Could you check a few things on this drawing? It's one solid part, dimensions in mm from its lowest x, y, z. A direction names the side the tool comes from. Give positions to 0.01 mm unless a question says otherwise; leave off trailing zeros. Order: outer loops, then holes, each group sorted by start corner. A loop starts at its lowest first (then second) coordinate and runs counter-clockwise, first axis right, second up. Notation, with made-up numbers: (3, 46) -> (40, 46) arc R20 cw to (40, 85) -> close; hole circle Ø11 at (86.25, 58.5). An arc over 180 degrees is marked (long way). Use one line per item in the form item = value. Start each with the question number.
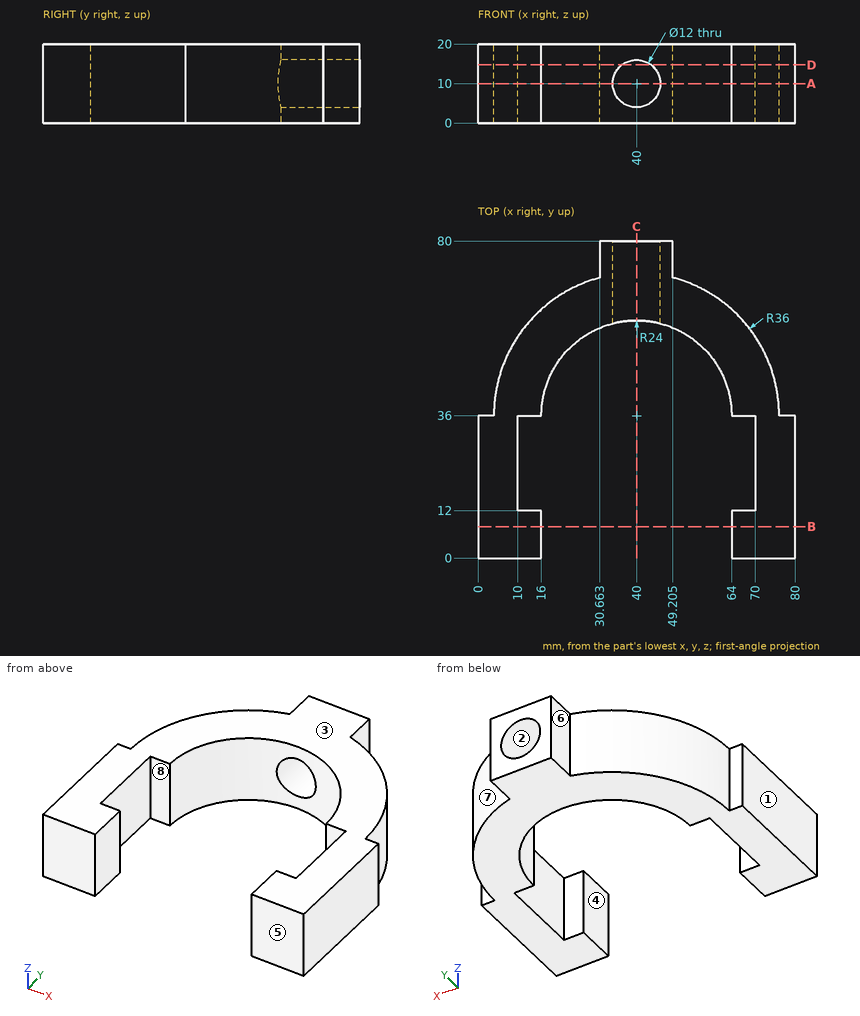
(1) Which directions (+Z, -Z, +X, -X, +Y, -Y) give clear straight access to the entire face, cutting with the end or side of a thin tool? Please do the marked faces 4, 5, 6, 7 and 8.
(2) Please list where these lines run through material, in increasing order: probe 1 along Z at (x, y) = (40, 71.5); probe 2 along X at (y, z) = (73.5, 10) (1 decimal); probe 3 along X at (y, z) = (24, 4.5).
(3) I'm going to push flat-ended pins straight in: pin 1 Ø2 at (x, z) = (78.5, 5.5) entering from +Y; pin 2 Ø10 at (y, z) = (74, 5.5) entering from +X (1 decimal); pin 3 Ø8 at (x, z) = (38, 6) entering from -Y. Where does each tip first touch, or does it pass through?
(4) Imagine slicing it at B-B (y = 8). Write out the boundary of the cut face in (x, z).
(5) We'd pull the mould along X, two halves only. Please class the marked faces 1, 2 and 3: pulls with the +X half, pulls with the -X half, needs draft (parallel to the pull), parting line crosses it, or undercut.
(6) Imagine slicing it at A-A (z = 10). Write out the boundary of the cut face in (x, y) (1 decimal).
(7) Imagine slicing it at C-C (x = 40). Write out the boundary of the cut face in (y, z), plus the area to 3 significant figures.
(8) Imagine slicing it at D-D (z = 14.75). Write out the boundary of the cut face in (x, y) (1 decimal), plus the area to 3 significant figures.
Calculated:
q1.face_4 = +Z, -Z, -Y
q1.face_5 = +Z, -Z, +X, -X, -Y
q1.face_6 = +Z, -Z, -X, +Y
q1.face_7 = +Z, -Z, +X, +Y
q1.face_8 = +Z, -Z
q2.probe_1 = 0 to 4, 16 to 20
q2.probe_2 = 30.7 to 34, 46 to 49.2
q2.probe_3 = 0 to 10, 70 to 80
q3.pin_1 = 36
q3.pin_2 = 54.4
q3.pin_3 = 59.24
q4.outline = (0, 0) -> (16, 0) -> (16, 20) -> (0, 20) -> close; (64, 0) -> (80, 0) -> (80, 20) -> (64, 20) -> close
q5.face_1 = pulls with the -X half
q5.face_2 = undercut
q5.face_3 = needs draft
q6.outline = (0, 0) -> (16, 0) -> (16, 12) -> (10, 12) -> (10, 36) -> (16, 36) arc R24 cw to (34, 59.2) -> (34, 80) -> (30.7, 80) -> (30.7, 70.8) arc R36 ccw to (4, 36) -> (0, 36) -> close; (46, 59.2) arc R24 cw to (64, 36) -> (70, 36) -> (70, 12) -> (64, 12) -> (64, 0) -> (80, 0) -> (80, 36) -> (76, 36) arc R36 ccw to (49.2, 70.8) -> (49.2, 80) -> (46, 80) -> close
q7.outline = (60, 0) -> (80, 0) -> (80, 4) -> (60, 4) -> close; (60, 16) -> (80, 16) -> (80, 20) -> (60, 20) -> close
q7.area = 160 mm2
q8.outline = (0, 0) -> (16, 0) -> (16, 12) -> (10, 12) -> (10, 36) -> (16, 36) arc R24 cw to (36.3, 59.7) -> (36.3, 80) -> (30.7, 80) -> (30.7, 70.8) arc R36 ccw to (4, 36) -> (0, 36) -> close; (43.7, 59.7) arc R24 cw to (64, 36) -> (70, 36) -> (70, 12) -> (64, 12) -> (64, 0) -> (80, 0) -> (80, 36) -> (76, 36) arc R36 ccw to (49.2, 70.8) -> (49.2, 80) -> (43.7, 80) -> close
q8.area = 2,000 mm2
